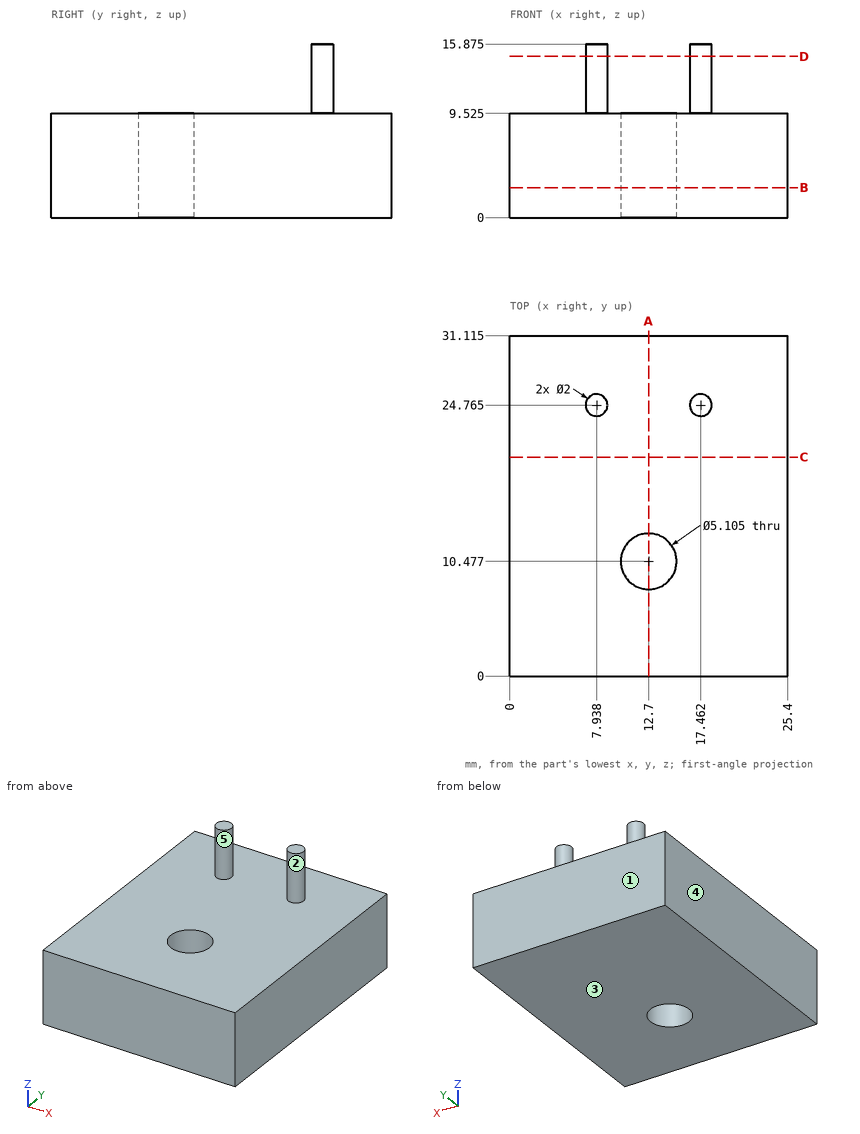
For this review, use the dimensioned drawing (mm, ordinates from the lowest corner) and the shaded views. A direction names the side the tool comes from. Give positions to 0.01 mm unless a question says otherwise; leave off trailing zeros. Order: outer loops, then holes, each group sorted by start corner. A loop starts at its lowest first (then second) coordinate and runs counter-clockwise, first axis right, second up.
1. Add section C-C, the plane y = 20. State the section outline as (x, z) points (1 decimal).
Solution:
outline: (0, 0) - (25.4, 0) - (25.4, 9.5) - (0, 9.5) - close
2. Add section A-A, the plane x = 12.7. State the section outline as (y, z) points (1 decimal).
Solution:
outline: (0, 0) - (7.9, 0) - (7.9, 9.5) - (0, 9.5) - close; (13, 0) - (31.1, 0) - (31.1, 9.5) - (13, 9.5) - close
3. Add section B-B, the plane z = 2.75. State the section outline as (x, y) points (1 decimal).
Solution:
outline: (0, 0) - (25.4, 0) - (25.4, 31.1) - (0, 31.1) - close; hole circle Ø5.1 at (12.7, 10.5)
4. To check wall thickness, follow L1, parallel to Y at x = 12.7, z = 4.5 (1 decimal); L2, parallel to Z at x = 17.5, y = 21 (1 decimal); L3, parallel to Y at x = 10.5, z = 4.75 (1 decimal). State the ranges of each line that lie inside material, in increasing order.
Solution:
L1: y = 0 to 7.9, 13 to 31.1
L2: z = 0 to 9.5
L3: y = 0 to 9.2, 11.8 to 31.1
5. Add section D-D, the plane z = 14.75. State the section outline as (x, y) points (1 decimal).
Solution:
outline: circle Ø2 at (7.9, 24.8); circle Ø2 at (17.5, 24.8)
6. Tool access review of the marked faces 1 and 2: name each direction out of +Z, -Z, +X, -X, +Y, -Y from which nothing blocks a thin tool from reaching the whole face with its end or side.
Solution:
face 1: +Z, -Z, +X, -X, +Y
face 2: +Z
7. Mouldability with a two-part tool opening along X and no side actions: class the marked faces 3, 4 and 5 as +X half, -X half, draft (parallel to the pull), parting line (faces both ways), or undercut.
Solution:
face 3: draft
face 4: -X half
face 5: undercut
8. For pin 1 Ø1 at (x, z) = (9, 11) entering from +Y; pin 2 Ø10 at (x, y) = (9.5, 7.5) entering from -Z; pin 3 Ø2 at (x, z) = (13.5, 13.5) entering from -Y; pin 4 Ø1.5 at (x, z) = (17.5, 12.5) entering from -Y (1 decimal), all flat-tipped, find the tip position at first contact; note any pin that passes through.
Solution:
pin 1: stops at y = 25.59
pin 2: stops at z = 0
pin 3: passes through
pin 4: stops at y = 23.8
